Read the model definition and answer for the solid it produces. Units are mm, in the model's axes. A direction names the side the tool comes from. Round coordinates to 2 decimals unless told otherwise and drop trailing zeros. Order: outer loops, then holes, each group sorted by start corner. A loop starts at its lowest first (then second) coordinate and runs counter-clockwise, first axis right, second up. Notation, with made-up numbers: (84, 17.25) - (96, 17.25) arc R15 ccw to (96, 45.25) - close; hole circle Ø6 at (43.25, -5). An arc over 180 degrees is marked (long way). Answer as a JSON object with one key per item and string values. Group by question number.
Q1. Given pin 1 Ø6 at (x, z) = (-20, 0) entering from +Y; pin 2 Ø2 at (y, z) = (13, 3.5) entering from +X; pin 3 Ø4 at (y, z) = (9, -1) entering from -X, each flat-ended and moving along its own axis, determine where each tip first touches the part or whether it passes through.
Q2. A cutting plane is placed at C-C on y = 1.5. Determine the outline of the cut face in (x, z), and give its area (3 significant figures).
Q3. A cutting plane is placed at B-B on y = 7.75. Determine the outline of the cut face in (x, z).
Q4. A cutting plane is placed at D-D on x = -20. Determine the outline of the cut face in (y, z).
Q5. The mould has two halves that part along X. Classify faces 5 (the cylindrical face through (-25, 2.54, 5.07)), 6 (the flat face through (6.5, 4, 0)), 7 (the conical face through (-7.3, 4.8, -0.1)): pulls with the +X half, pulls with the -X half, needs draft (parallel to the pull), parting line crosses it, or undercut.
Q6. Consider line 1 (Z direction, x = 0, y = 14.5); line 2 (Z direction, x = -20, y = 1.95); line 3 (Y direction, x = -5, z = -4.25). Determine where each line is inside the solid, lowest interval first.
Q7. A cutting plane is placed at A-A on x = 0. Determine the outline of the cut face in (y, z), and give its area (3 significant figures).
Q8. A tool of negligible diameter and unlimited length cuts with its end or side. For faces 1 (the cylindrical face through (-8.65, 2.03, -0.07)), 2 (the flat face through (-2, 9, 6)), 3 (the cylindrical face through (-5.07, 7.03, -5)), 4 (the cylindrical face through (-5.07, 7.03, 5)), from which of +Z, -Z, +X, -X, +Y, -Y can it reach the whole face along a straight path? Write none if from no direction.
```python
from build123d import *

# Parameters (mm, degrees)
SKETCH_1_W             = 33
SKETCH_1_H             = 13
SKETCH_1_R             = 2.23020675
EXTRUDE_1_DEPTH        = 5
SKETCH_1_5_R           = 6
EXTRUDE_2_DEPTH        = 20
HOLE_WIZARD_M6_1_D     = 5
HOLE_WIZARD_M6_2_D     = 5
SKETCH_10_W            = 13
SKETCH_10_H            = 13
SKETCH_10_R            = 6
EXTRUDE_3_DEPTH        = 4
HOLE_WIZARD_M4_1_D     = 3.3
HOLE_WIZARD_M4_1_DEPTH = 4
HOLE_WIZARD_M4_1_TIP   = 0.991420021
FILLET_1_R             = 5


with BuildPart() as part:
    # 草图1 → 凸台-拉伸1 (new body)
    with BuildSketch(Plane(origin=(0, 0, 0), x_dir=(1, 0, 0), z_dir=(0, 1, 0))):
        with Locations((-10, 0)):
            Rectangle(SKETCH_1_W, SKETCH_1_H)
        with Locations((-20, 0)):
            Circle(SKETCH_1_R, mode=Mode.SUBTRACT)
    extrude(amount=EXTRUDE_1_DEPTH)

    # 草图1<5> → 凸台-拉伸2 (add)
    with BuildSketch(Plane(origin=(0, 0, 0), x_dir=(1, 0, 0), z_dir=(0, 1, 0))):
        Circle(SKETCH_1_5_R)
    extrude(amount=EXTRUDE_2_DEPTH)

    # M6 螺纹孔1 (through all)
    with Locations(Plane(origin=(0, 20, 0), x_dir=(1, 0, 0), z_dir=(0, 1, 0))):
        with Locations((0, 0)):
            Hole(HOLE_WIZARD_M6_1_D / 2)

    # M6 螺纹孔2 (through all)
    with Locations(Plane(origin=(0, 5, 0), x_dir=(1, 0, 0), z_dir=(0, 1, 0))):
        with Locations((-20, 0)):
            Hole(HOLE_WIZARD_M6_2_D / 2)

    # 草图10 → 凸台-拉伸3 (add)
    with BuildSketch(Plane(origin=(0, 5, 0), x_dir=(1, 0, 0), z_dir=(0, 1, 0))):
        Rectangle(SKETCH_10_W, SKETCH_10_H)
        Circle(SKETCH_10_R, mode=Mode.SUBTRACT)
    extrude(amount=EXTRUDE_3_DEPTH)

    # M4 螺纹孔1
    with Locations(Plane(origin=(0, 0, 0), x_dir=(-1, 0, 0), z_dir=(0, -1, 0))):
        with Locations((7, 0)):
            Hole(HOLE_WIZARD_M4_1_D / 2, depth=HOLE_WIZARD_M4_1_DEPTH)
            with Locations((0, 0, -(HOLE_WIZARD_M4_1_DEPTH + HOLE_WIZARD_M4_1_TIP / 2))):  # 118° drill point
                Cone(0, HOLE_WIZARD_M4_1_D / 2, HOLE_WIZARD_M4_1_TIP, mode=Mode.SUBTRACT)

    # 圆角1
    fillet_1_edges = [part.edges().sort_by_distance(p)[0] for p in [
        (-26.5, 2.5, 6.5),
        (-26.5, 2.5, -6.5),
        (6.5, 4.5, -6.5),
        (6.5, 4.5, 6.5),
        (-6.5, 7, -6.5),
        (-6.5, 7, 6.5),
    ]]
    fillet(fillet_1_edges, radius=FILLET_1_R)


solid = part.part
```
Result set:
{
 "1": {"pin 1": "stops at y = 5", "pin 2": "stops at x = 5.45", "pin 3": "stops at x = -6.5"},
 "2": {"outline": "(-26.5, -1.5) arc R5 ccw to (-21.5, -6.5) - (1.5, -6.5) arc R5 ccw to (6.5, -1.5) - (6.5, 1.5) arc R5 ccw to (1.5, 6.5) - (-21.5, 6.5) arc R5 ccw to (-26.5, 1.5) - close; hole circle Ø5 at (-20, 0); hole circle Ø3.3 at (-7, 0); hole circle Ø5 at (0, 0)", "area": "360 mm²"},
 "3": {"outline": "(-6.5, -1.5) arc R5 ccw to (-1.5, -6.5) - (1.5, -6.5) arc R5 ccw to (6.5, -1.5) - (6.5, 1.5) arc R5 ccw to (1.5, 6.5) - (-1.5, 6.5) arc R5 ccw to (-6.5, 1.5) - close; hole circle Ø5 at (0, 0)"},
 "4": {"outline": "(0, -6.5) - (5, -6.5) - (5, -2.5) - (0, -2.5) - close; (0, 2.5) - (5, 2.5) - (5, 6.5) - (0, 6.5) - close"},
 "5": {"face 5": "pulls with the -X half", "face 6": "pulls with the +X half", "face 7": "undercut"},
 "6": {"line 1": "z = -6 to -2.5, 2.5 to 6", "line 2": "z = -6.5 to -2.5, 2.5 to 6.5", "line 3": "y = 0 to 9"},
 "7": {"outline": "(0, -6.5) - (9, -6.5) - (9, -6) - (20, -6) - (20, -2.5) - (0, -2.5) - close; (0, 2.5) - (20, 2.5) - (20, 6) - (9, 6) - (9, 6.5) - (0, 6.5) - close", "area": "149 mm²"},
 "8": {"face 1": "-Y", "face 2": "+Y", "face 3": "-Z, -X, +Y", "face 4": "+Z, -X, +Y"}
}
